Input: part model. Units: mm. Frame: model coordinates. A direction names the side the tool comes from. Round coordinates to 2 decimals unless told otherwise and drop trailing zeros. Loops run counter-clockwise (first coordinate to the right, second up) from the corner with the lowest first, then second, coordinate; pieces in that order, holes last. Notation, with made-up numbers: (47.5, 14) -> (99.5, 14) arc R17 cw to (99.5, 33) -> close; hole circle Ø2 at (55.5, 40). An arc over 180 degrees is marked (long way). Answer as a JSON object with one key per item and string values.
```python
from build123d import *

# Parameters (mm, degrees)
F0_R     = 10
F1_DEPTH = 25
F2_D     = 7.9375
F2_DEPTH = 22
F2_TIP   = 2.3846655818


with BuildPart() as f1:
    # F0 (on Top) → F1 (new body)
    with BuildSketch(Plane.XY):
        Circle(F0_R)
    extrude(amount=F1_DEPTH)

    # F2
    with Locations(Plane(origin=(0, 0, 0), x_dir=(1, 0, 0), z_dir=(0, 0, -1))):
        with Locations((0, 0)):
            Hole(F2_D / 2, depth=F2_DEPTH)
            with Locations((0, 0, -(F2_DEPTH + F2_TIP / 2))):  # 118° drill point
                Cone(0, F2_D / 2, F2_TIP, mode=Mode.SUBTRACT)

    # F3 (on Front) → F4 (revolve, cut)
    with BuildSketch(Plane.XZ):
        Polygon((-10, 11), (-10, 0), (-9, 0), align=None)
    revolve(axis=Axis((0, 0, 5.5), (0, 0, 1)), mode=Mode.SUBTRACT)


solid = f1.part
```
1) Reachability of faces 4 (the face through (-2.17, -9.76, 17.9)), 5 (the face through (0.86, 3.874, 11.154)) from +Z, -Z, +X, -X, +Y, -Y: full face, straight path, thin tool, end or side. Return the list, or none.
Output:
{"face 4": "+Z, -Z", "face 5": "-Z"}
2) Ray query, probe 1 along Y at (x, z) = (0, 15.5); probe 2 along Y at (x, z) = (-2.75, 10.75); probe 3 along Y at (x, z) = (7.25, 12.75). Return the intervals inside material, ascending.
Output:
{"probe 1": "y = -10 to -3.97, 3.97 to 10", "probe 2": "y = -9.59 to -2.86, 2.86 to 9.59", "probe 3": "y = -6.89 to 6.89"}
3) Section A-A, the plane z = 14.25. Output: boundary loops of the cut face in (x, y).
Output:
{"outline": "circle Ø20 at (0, 0); hole circle Ø7.94 at (0, 0)"}
4) Contact query for flat-ended pins moving along their axis: P1, Ø8, axis at x = 6.5, z = 20, coming from the -Y side; P2, Ø4, axis at x = 5.5, z = 8, coming from the -Y side; P3, Ø2, axis at x = -2.5, z = 15, coming from the +Y side. Output: stop coordinate, or through.
Output:
{"P1": "stops at y = -9.68", "P2": "stops at y = -9.1", "P3": "stops at y = 9.89"}
5) Section B-B, the plane z = 8.25. Output: boundary loops of the cut face in (x, y).
Output:
{"outline": "circle Ø19.5 at (0, 0); hole circle Ø7.94 at (0, 0)"}
6) Draft query along X for faces 1 (the face through (-0.51, -0.47, 23.97)), 2 (the face through (-8.962, -2.822, 4.355)), 3 (the face through (2, -4, 0)). Return one class per face: +X half, -X half, draft (parallel to the pull), parting line (faces both ways), or undercut.
Output:
{"face 1": "undercut", "face 2": "parting line", "face 3": "draft"}
